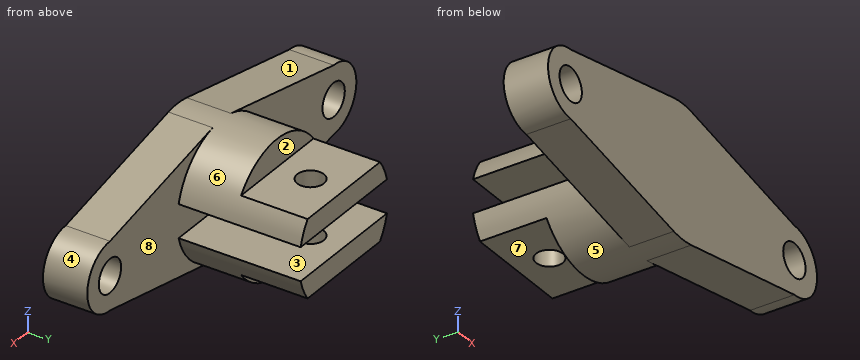
from build123d import *

# Parameters (mm, degrees)
CROQUIS2_R                 = 7.5
SALIENTE_EXTRUIR1_DEPTH    = 20
SALIENTE_EXTRUIR2_START    = 20
SALIENTE_EXTRUIR2_DEPTH    = 25
SALIENTE_EXTRUIR3_START    = 45
SALIENTE_EXTRUIR3_DEPTH    = 30
CORTAR_EXTRUIR1_DEPTH      = 122.287306133
CORTAR_EXTRUIR1_DEPTH_BACK = 122.287306133
CROQUIS4_R                 = 6


with BuildPart() as part:
    # Croquis2 → Saliente-Extruir1 (new body)
    # profile 1 of 5: a face of its own
    with BuildSketch(Plane(origin=(0, 0, 0), x_dir=(1, 0, 0), z_dir=(0, 1, 0))):
        with BuildLine():
            ThreePointArc((-75.223489404, 15.549419201), (-90.474364485, 0.29854412), (-75.223489404, -14.952330962))
            Line((-75.223489404, -14.952330962), (-6.126869665, -29.367694293))
            ThreePointArc((-6.126869665, -29.367694293), (-16.360909149, -25.145986793), (-24.366985862, -17.5))
            ThreePointArc((-24.366985862, -17.5), (-27.171188586, -12.717173855), (-29.047375097, -7.5))
            Line((-29.047375097, -7.5), (29.047375097, -7.5))
            ThreePointArc((29.047375097, -7.5), (27.171188586, -12.717173855), (24.366985862, -17.5))
            ThreePointArc((24.366985862, -17.5), (16.360909149, -25.145986793), (6.126869665, -29.367694293))
            Line((6.126869665, -29.367694293), (75.223489404, -14.952330962))
            ThreePointArc((75.223489404, -14.952330962), (90.474364485, 0.29854412), (75.223489404, 15.549419201))
            Line((75.223489404, 15.549419201), (5.883484054, 29.417420271))
            ThreePointArc((5.883484054, 29.417420271), (16.256658913, 25.213509097), (24.366985862, 17.5))
            ThreePointArc((24.366985862, 17.5), (27.171188586, 12.717173855), (29.047375097, 7.5))
            Line((29.047375097, 7.5), (-29.047375097, 7.5))
            ThreePointArc((-29.047375097, 7.5), (-27.171188586, 12.717173855), (-24.366985862, 17.5))
            ThreePointArc((-24.366985862, 17.5), (-16.256658913, 25.213509097), (-5.883484054, 29.417420271))
            Line((-5.883484054, 29.417420271), (-75.223489404, 15.549419201))
        make_face()
        with Locations(Location((-75.223489404, 0.29854412, 0), (0, 0, 270))):
            Circle(CROQUIS2_R, mode=Mode.SUBTRACT)
        with Locations(Location((75.223489404, 0.29854412, 0), (0, 0, 270))):
            Circle(CROQUIS2_R, mode=Mode.SUBTRACT)
    # profile 2 of 5: a face of its own
    with BuildSketch(Plane(origin=(0, 0, 0), x_dir=(1, 0, 0), z_dir=(0, 1, 0))):
        with BuildLine():
            ThreePointArc((-24.366985862, -17.5), (-16.360909149, -25.145986793), (-6.126869665, -29.367694293))
            ThreePointArc((-6.126869665, -29.367694293), (0, -30), (6.126869665, -29.367694293))
            ThreePointArc((6.126869665, -29.367694293), (16.360909149, -25.145986793), (24.366985862, -17.5))
            Line((24.366985862, -17.5), (-24.366985862, -17.5))
        make_face()
    # profile 3 of 5: a face of its own
    with BuildSketch(Plane(origin=(0, 0, 0), x_dir=(1, 0, 0), z_dir=(0, 1, 0))):
        with BuildLine():
            ThreePointArc((-29.047375097, -7.5), (-27.171188586, -12.717173855), (-24.366985862, -17.5))
            Line((-24.366985862, -17.5), (24.366985862, -17.5))
            ThreePointArc((24.366985862, -17.5), (27.171188586, -12.717173855), (29.047375097, -7.5))
            Line((29.047375097, -7.5), (-29.047375097, -7.5))
        make_face()
    # profile 4 of 5: a face of its own
    with BuildSketch(Plane(origin=(0, 0, 0), x_dir=(1, 0, 0), z_dir=(0, 1, 0))):
        with BuildLine():
            Line((24.366985862, 17.5), (-24.366985862, 17.5))
            ThreePointArc((-24.366985862, 17.5), (-27.171188586, 12.717173855), (-29.047375097, 7.5))
            Line((-29.047375097, 7.5), (29.047375097, 7.5))
            ThreePointArc((29.047375097, 7.5), (27.171188586, 12.717173855), (24.366985862, 17.5))
        make_face()
    # profile 5 of 5: a face of its own
    with BuildSketch(Plane(origin=(0, 0, 0), x_dir=(1, 0, 0), z_dir=(0, 1, 0))):
        with BuildLine():
            ThreePointArc((5.883484054, 29.417420271), (0, 30), (-5.883484054, 29.417420271))
            ThreePointArc((-5.883484054, 29.417420271), (-16.256658913, 25.213509097), (-24.366985862, 17.5))
            Line((-24.366985862, 17.5), (24.366985862, 17.5))
            ThreePointArc((24.366985862, 17.5), (16.256658913, 25.213509097), (5.883484054, 29.417420271))
        make_face()
    extrude(amount=SALIENTE_EXTRUIR1_DEPTH)

    # Croquis2<3> → Saliente-Extruir2 (add)
    with BuildSketch(Plane(origin=(0, 0, 0), x_dir=(1, 0, 0), z_dir=(0, 1, 0)).offset(SALIENTE_EXTRUIR2_START)):
        with BuildLine():
            ThreePointArc((-24.366985862, -17.5), (-16.360909149, -25.145986793), (-6.126869665, -29.367694293))
            ThreePointArc((-6.126869665, -29.367694293), (0, -30), (6.126869665, -29.367694293))
            ThreePointArc((6.126869665, -29.367694293), (16.360909149, -25.145986793), (24.366985862, -17.5))
            Line((24.366985862, -17.5), (-24.366985862, -17.5))
        make_face()
        with BuildLine():
            ThreePointArc((-29.047375097, -7.5), (-27.171188586, -12.717173855), (-24.366985862, -17.5))
            Line((-24.366985862, -17.5), (24.366985862, -17.5))
            ThreePointArc((24.366985862, -17.5), (27.171188586, -12.717173855), (29.047375097, -7.5))
            Line((29.047375097, -7.5), (-29.047375097, -7.5))
        make_face()
        with BuildLine():
            Line((24.366985862, 17.5), (-24.366985862, 17.5))
            ThreePointArc((-24.366985862, 17.5), (-27.171188586, 12.717173855), (-29.047375097, 7.5))
            Line((-29.047375097, 7.5), (29.047375097, 7.5))
            ThreePointArc((29.047375097, 7.5), (27.171188586, 12.717173855), (24.366985862, 17.5))
        make_face()
        with BuildLine():
            ThreePointArc((5.883484054, 29.417420271), (0, 30), (-5.883484054, 29.417420271))
            ThreePointArc((-5.883484054, 29.417420271), (-16.256658913, 25.213509097), (-24.366985862, 17.5))
            Line((-24.366985862, 17.5), (24.366985862, 17.5))
            ThreePointArc((24.366985862, 17.5), (16.256658913, 25.213509097), (5.883484054, 29.417420271))
        make_face()
    extrude(amount=SALIENTE_EXTRUIR2_DEPTH)

    # Croquis2<4> → Saliente-Extruir3 (add)
    with BuildSketch(Plane(origin=(0, 0, 0), x_dir=(1, 0, 0), z_dir=(0, 1, 0)).offset(SALIENTE_EXTRUIR3_START)):
        with BuildLine():
            ThreePointArc((-29.047375097, -7.5), (-27.171188586, -12.717173855), (-24.366985862, -17.5))
            Line((-24.366985862, -17.5), (24.366985862, -17.5))
            ThreePointArc((24.366985862, -17.5), (27.171188586, -12.717173855), (29.047375097, -7.5))
            Line((29.047375097, -7.5), (-29.047375097, -7.5))
        make_face()
        with BuildLine():
            Line((24.366985862, 17.5), (-24.366985862, 17.5))
            ThreePointArc((-24.366985862, 17.5), (-27.171188586, 12.717173855), (-29.047375097, 7.5))
            Line((-29.047375097, 7.5), (29.047375097, 7.5))
            ThreePointArc((29.047375097, 7.5), (27.171188586, 12.717173855), (24.366985862, 17.5))
        make_face()
    extrude(amount=SALIENTE_EXTRUIR3_DEPTH)

    # Croquis4 → Cortar-Extruir1 (cut, two sides: drawn at the far end of the back side and taken through both)
    with BuildSketch(Plane.XY.offset(-CORTAR_EXTRUIR1_DEPTH_BACK)):
        with Locations((0, 60)):
            Circle(CROQUIS4_R)
    extrude(amount=CORTAR_EXTRUIR1_DEPTH + CORTAR_EXTRUIR1_DEPTH_BACK, mode=Mode.SUBTRACT)


solid = part.part
Geometry check sheet. Reference: the model listing, model coordinates, mm. Face numbers are marked on the shaded views. A direction names the side the tool comes from. Give positions to 0.01 mm unless a question says otherwise; leave off trailing zeros. Order: outer loops, then holes, each group sorted by start corner. A loop starts at its lowest first (then second) coordinate and runs counter-clockwise, first axis right, second up.
1. Draft check along Z on the marked faces 6, 7 and 8. Enter one of: pulls with the +Z half, pulls with the -Z half, needs draft (parallel to the pull), parting line crosses it, or undercut.
Completed:
face 6: pulls with the +Z half
face 7: pulls with the -Z half
face 8: undercut
2. Scan lines: line 1 (Y direction, x = 0, z = 14.5); line 2 (Z direction, x = -24, y = 53); line 3 (Y direction, x = -26, z = 15.5). Record each from-to range of solid material in increasing order.
Completed:
line 1: y = 0 to 54, 66 to 75
line 2: z = -17.5 to -7.5, 7.5 to 17.5
line 3: y = 0 to 20
3. Sectioned sample at C-C (y = 60). Record the boundary of the cut face in (x, z), then the cut area to 3 significant figures.
Completed:
outline: (-29.05, -7.5) arc R30 ccw to (-24.37, -17.5) - (-6, -17.5) - (-6, -7.5) - close; (-29.05, 7.5) - (-6, 7.5) - (-6, 17.5) - (-24.37, 17.5) arc R30 ccw to start; (6, -17.5) - (24.37, -17.5) arc R30 ccw to (29.05, -7.5) - (6, -7.5) - close; (6, 7.5) - (29.05, 7.5) arc R30 ccw to (24.37, 17.5) - (6, 17.5) - close
area: 843 mm2
4. Depth check by flat-ended pin: pin 1 (14 mm diameter, centred on x = 0, y = 60, fed in from +Z); pin 2 (3 mm diameter, centred on y = 30, z = -16, fed in from -X); pin 3 (9.5 mm diameter, centred on x = 0, y = 60, fed in from +Z) (3 decimals); pin 4 (8 mm diameter, centred on x = 4.5, y = 13, fed in from +Z). Enter the tip coordinate at first touch or a pass-through.
Completed:
pin 1: stops at z = 17.5
pin 2: stops at x = -26.26
pin 3: passes through
pin 4: stops at z = 30
5. Access from +Z, -Z, +X, -X, +Y, -Y to the whole of each face (thin tool, end or side, straight path). Record for the marked faces 1, 2, 3, 4 and 5.
Completed:
face 1: +Z, -X, +Y, -Y
face 2: +Z, +X, -X, +Y
face 3: +X, -X, +Y
face 4: +X, +Y, -Y
face 5: -Z, +Y
6. Sectioned sample at B-B (x = 0). Record the boundary of the cut face in (y, z), then the cut area to 4 significant figures.
Completed:
outline: (0, -30) - (45, -30) - (45, -17.5) - (54, -17.5) - (54, -7.5) - (20, -7.5) - (20, 7.5) - (54, 7.5) - (54, 17.5) - (45, 17.5) - (45, 30) - (0, 30) - close; (66, -17.5) - (75, -17.5) - (75, -7.5) - (66, -7.5) - close; (66, 7.5) - (75, 7.5) - (75, 17.5) - (66, 17.5) - close
area: 2,685 mm2
7. Sectioned sample at A-A (y = 50.5). Record the boundary of the cut face in (x, z).
Completed:
outline: (-29.05, -7.5) arc R30 ccw to (-24.37, -17.5) - (24.37, -17.5) arc R30 ccw to (29.05, -7.5) - close; (-29.05, 7.5) - (29.05, 7.5) arc R30 ccw to (24.37, 17.5) - (-24.37, 17.5) arc R30 ccw to start
8. Sectioned sample at D-D (z = -12.5). Record the boundary of the cut face in (x, y), then the cut area to 3 significant figures.
Completed:
outline: (-84.37, 0) - (84.37, 0) - (84.37, 20) - (27.27, 20) - (27.27, 75) - (-27.27, 75) - (-27.27, 20) - (-84.37, 20) - close; hole circle Ø12 at (0, 60)
area: 6,260 mm2
